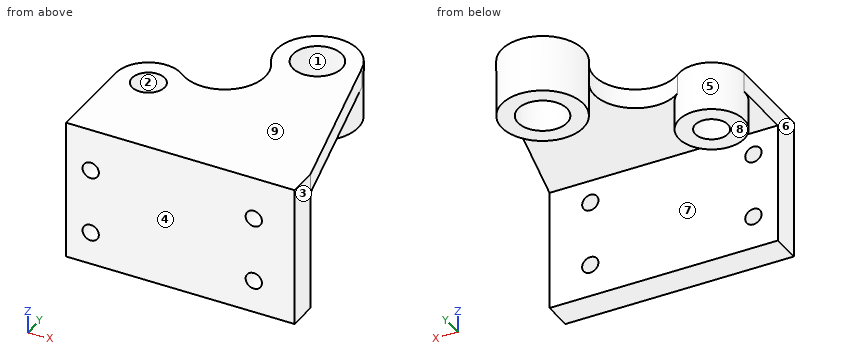
from build123d import *

# Parameters (mm, degrees)
SKETCH1_W            = 140
SKETCH1_H            = 86
BOSS_EXTRUDE1_DEPTH  = 18
BOSS_EXTRUDE2_DEPTH  = 12
SKETCH2_4_R          = 25
SKETCH2_4_R_2        = 15
BOSS_EXTRUDE3_DEPTH  = 35
SKETCH2_6_R          = 20
SKETCH2_6_R_2        = 10
BOSS_EXTRUDE4_DEPTH  = 30
HOLE1_OUTLINE_R      = 5
HOLE1_DEPTH          = 18
LPATTERN1_COUNT      = 2
LPATTERN1_PITCH      = 100
LPATTERN1_COUNT_DIR2 = 2
LPATTERN1_PITCH_DIR2 = 40


# Read off the part's stored shape, not the designer's step: Hole1
with BuildPart() as part:
    # Sketch1 → Boss-Extrude1 (new body)
    with BuildSketch(Plane(origin=(0, 0, 0), x_dir=(1, 0, 0), z_dir=(0, 1, 0))):
        Rectangle(SKETCH1_W, SKETCH1_H)
    extrude(amount=BOSS_EXTRUDE1_DEPTH)

    # Sketch2 → Boss-Extrude2 (add)
    with BuildSketch(Plane.XY.offset(43)):
        with BuildLine():
            ThreePointArc((-30, 56), (-50, 36), (-70, 56))
            Line((-70, 56), (-70, 18))
            Line((-70, 18), (70, 18))
            Line((70, 18), (44.294494718, 123.897247359))
            ThreePointArc((44.294494718, 123.897247359), (44.822997079, 120.969649142), (45, 118))
            ThreePointArc((45, 118), (26.869042098, 93.962191018), (-1.225300853, 104.790662253))
            ThreePointArc((-1.225300853, 104.790662253), (-5.698641076, 73.02406676), (-37.75582298, 71.813922003))
            ThreePointArc((-37.75582298, 71.813922003), (-32.043336329, 64.80671504), (-30, 56))
        make_face()
    extrude(amount=-BOSS_EXTRUDE2_DEPTH)

    # Sketch2<4> → Boss-Extrude3 (add)
    with BuildSketch(Plane.XY.offset(43)):
        with Locations((20, 118)):
            Circle(SKETCH2_4_R)
        with Locations((20, 118)):
            Circle(SKETCH2_4_R_2, mode=Mode.SUBTRACT)
    extrude(amount=-BOSS_EXTRUDE3_DEPTH)

    # Sketch2<6> → Boss-Extrude4 (add)
    with BuildSketch(Plane.XY.offset(43)):
        with Locations((-50, 56)):
            Circle(SKETCH2_6_R)
        with Locations((-50, 56)):
            Circle(SKETCH2_6_R_2, mode=Mode.SUBTRACT)
    extrude(amount=-BOSS_EXTRUDE4_DEPTH)

    # Hole1 outline → Hole1 (cut)
    with BuildSketch(Plane(origin=(0, 0, 0), x_dir=(1, 0, 0), z_dir=(0, 1, 0))):
        with Locations((-55, 23)):
            Circle(HOLE1_OUTLINE_R)
    hole1 = extrude(amount=HOLE1_DEPTH, mode=Mode.SUBTRACT)

    # LPattern1: Hole1 2 × 2
    with Locations(*[(i * LPATTERN1_PITCH, 0, j * LPATTERN1_PITCH_DIR2) for i in range(LPATTERN1_COUNT) for j in range(LPATTERN1_COUNT_DIR2) if (i, j) != (0, 0)]):
        add(hole1, mode=Mode.SUBTRACT)


solid = part.part
Geometry check sheet. Reference: the model listing, model coordinates, mm. Face numbers are marked on the shaded views. A direction names the side the tool comes from. Give positions to 0.01 mm unless a question says otherwise; leave off trailing zeros. Write each loop counter-clockwise with the first axis right and the second up, starting at its lowest first coordinate (ties: lowest second). Pieces come first, ordered by that corner, then holes. Notation, with made-up numbers: M 62,-8 L 116,-8 A7 cw 116,2 Z; hole C 18.5,75.5 d10. An arc over 180 degrees is marked long. Answer as CSV lines item,"result". Start each with the question number.
Q1. Tool access check on the marked faces 5, 6, 7, 8 and 9. Record the directions out of +Z, -Z, +X, -X, +Y, -Y that give a thin tool (end or side, any length) a straight path to the whole face; none if there is none.
Q2. Section check D-D, the plane z = 6. Record the cut outline in (x, y), then the cut area to 3 significant figures.
Q3. Release check for a two-part mould opening along X. For the marked faces 1, 2, 3 and 4 record: pulls with the +X half, pulls with the -X half, needs draft (parallel to the pull), parting line crosses it, or undercut.
Q4. Go/stop test with flat-tipped pins: pin 1 (3 mm diameter, centred on y = 127, z = 16, fed in from +X); pin 2 (9 mm diameter, centred on x = 45, z = 17, fed in from +Y); pin 3 (3 mm diameter, centred on x = 8.5, y = 20, fed in from -Z). Record where each tip stops, or that it passes through.
Q5. Material ranges on L1, parallel to Y at x = -50, z = 25.75; L2, parallel to Y at x = 20, z = 17; L3, parallel to X at y = 9.25, z = -23, recorded low to high.
Q6. Section check B-B, the plane x = -55. Record the cut outline in (y, z).
Q7. Section check A-A, the plane z = 17. Record the cut outline in (x, y).
Q8. Section check C-C, the plane y = 98.5. Record the cut outline in (x, z), then the cut area to 3 significant figures.
Geometry says:
1,face 5,"-Z"
1,face 6,"+Z, -Z, -X, +Y, -Y"
1,face 7,"-Z, +X, -X"
1,face 8,"-Z, +X, -X, +Y"
1,face 9,"+Z, +X, -X, +Y, -Y"
2,outline,"M -70,0 L 70,0 L 70,18 L -70,18 Z"
2,area,"2,520 mm^2"
3,face 1,"undercut"
3,face 2,"undercut"
3,face 3,"pulls with the +X half"
3,face 4,"needs draft"
4,pin 1,"x = 43.85"
4,pin 2,"y = 132.31"
4,pin 3,"z = 31"
5,L1,"0 to 18, 36 to 46, 66 to 76"
5,L2,"0 to 18, 93 to 103, 133 to 143"
5,L3,"-70 to -60, -50 to 40, 50 to 70"
6,outline,"M 0,-43 L 18,-43 L 18,-28 L 0,-28 Z; M 0,-18 L 18,-18 L 18,12 L 0,12 Z; M 0,22 L 18,22 L 18,31 L 36.64,31 L 36.64,13 L 47.34,13 L 47.34,43 L 0,43 Z; M 64.66,13 L 75.36,13 L 75.36,43 L 64.66,43 Z"
7,outline,"M -70,0 L -60,0 L -60,18 L -70,18 Z; C -50,56 d40; M -50,0 L 40,0 L 40,18 L -50,18 Z; C 20,118 d50; M 50,0 L 70,0 L 70,18 L 50,18 Z; hole C -50,56 d20; hole C 20,118 d30"
8,outline,"M 1.57,31 L 4.36,31 L 4.36,8 L 35.64,8 L 35.64,31 L 50.46,31 L 50.46,43 L 1.57,43 Z"
8,area,"1,310 mm^2"
